Source: CAD feature listing. Evaluate the final solid. Frame: model axes, mm. Give positions to 0.01 mm unless a question says otherwise; leave off trailing zeros. Order: outer loops, then holes, each group sorted by start corner. A loop starts at its lowest first (then second) coordinate and runs counter-clockwise, first axis right, second up.
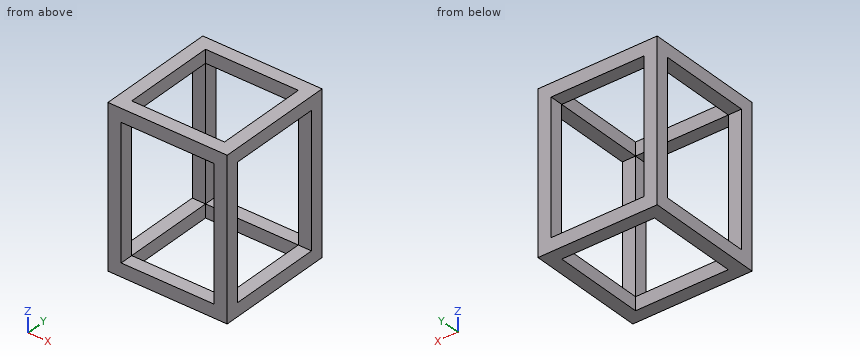
```python
from build123d import *

# Parameters (mm, degrees)
F0_W     = 914.4
F0_H     = 1219.2
F0_W_2   = 711.2
F0_H_2   = 1016
F1_DEPTH = 914.4
F2_W     = 711.2
F2_H     = 711.2
F3_DEPTH = 1219.2
F4_W     = 711.2
F4_H     = 1016
F5_DEPTH = 914.4


with BuildPart() as f1:
    # F0 (on Front) → F1 (new body)
    with BuildSketch(Plane.XZ):
        Rectangle(F0_W, F0_H)
        Rectangle(F0_W_2, F0_H_2, mode=Mode.SUBTRACT)
    extrude(amount=-F1_DEPTH)

    # F2 (on face) → F3 (cut)
    with BuildSketch(Plane.XY.offset(609.6)):
        with Locations((0, 457.2)):
            Rectangle(F2_W, F2_H)
    extrude(amount=-F3_DEPTH, mode=Mode.SUBTRACT)

    # F4 (on face) → F5 (cut)
    with BuildSketch(Plane(origin=(-457.2, 0, 0), x_dir=(0, -1, 0), z_dir=(-1, 0, 0))):
        with Locations((-457.2, 0)):
            Rectangle(F4_W, F4_H)
    extrude(amount=-F5_DEPTH, mode=Mode.SUBTRACT)


solid = f1.part
```
1) Section query B-B, the plane y = 378. Return the cut outline in (x, z).
Report:
outline: (-457.2, -609.6) - (-355.6, -609.6) - (-355.6, -508) - (-457.2, -508) - close; (-457.2, 508) - (-355.6, 508) - (-355.6, 609.6) - (-457.2, 609.6) - close; (355.6, -609.6) - (457.2, -609.6) - (457.2, -508) - (355.6, -508) - close; (355.6, 508) - (457.2, 508) - (457.2, 609.6) - (355.6, 609.6) - close
2) Material intervals for L1, parallel to Z at x = -416, y = 191.5; L2, parallel to X at y = 853, z = 67; L3, parallel to Y at x = 379.5, z = 28, sorted ascending.
Report:
L1: z = -609.6 to -508, 508 to 609.6
L2: x = -457.2 to -355.6, 355.6 to 457.2
L3: y = 0 to 101.6, 812.8 to 914.4
3) Section query A-A, the plane x = 15. Return the cut outline in (y, z), and give its area (3 significant figures).
Report:
outline: (0, -609.6) - (101.6, -609.6) - (101.6, -508) - (0, -508) - close; (0, 508) - (101.6, 508) - (101.6, 609.6) - (0, 609.6) - close; (812.8, -609.6) - (914.4, -609.6) - (914.4, -508) - (812.8, -508) - close; (812.8, 508) - (914.4, 508) - (914.4, 609.6) - (812.8, 609.6) - close
area: 41,300 mm2
4) Section query C-C, the plane x = -372. Return the cut outline in (y, z), and give its area (3 significant figures).
Report:
outline: (0, -609.6) - (914.4, -609.6) - (914.4, 609.6) - (0, 609.6) - close; hole (101.6, -508) - (812.8, -508) - (812.8, 508) - (101.6, 508) - close
area: 392,000 mm2
